Verification items for the finished model (mm, model axes). A direction names the side the tool comes from. Coordinates: 2 decimals unless noted, no trailing zeros. Order: outer loops, then holes, each group sorted by start corner. A loop starts at its lowest first (then second) coordinate and runs counter-clockwise, first axis right, second up.
Q1. Cross-section at D-D, the plane y = 9. Record the boundary of the cut face in (x, z).
Q2. Cross-section at C-C, the plane z = 15.5. Record the boundary of the cut face in (x, y).
Q3. Cross-section at B-B, the plane x = 2.5. Record the boundary of the cut face in (y, z).
Q4. Depth check by flat-ended pin: P1, Ø9.5, axis at y = 5, z = 17, coming from the +X side; P2, Ø6, axis at x = 4, y = 3, coming from the +Z side; P3, Ø10, axis at x = -4, y = -1, coming from the +Z side. Enter the tip coordinate at first touch or a pass-through.
Q5. Set-up check for faces 1 (the flat face through (-10, 6, 23.5)), 2 (the flat face through (0, -0.24, 10)): record each of +Z, -Z, +X, -X, +Y, -Y from which the full face is reachable in a straight line by a thin tool's end or side.
Q6. Cross-section at A-A, the plane y = 5.76. Record the boundary of the cut face in (x, z).
Q7. Draft check along X on faces 3 (the flat face through (-2, -3.24, 9)), 4 (the cylindrical face through (2.35, 4.24, 1.77)), 5 (the flat face through (-8.178, 5.634, 22.514)). Enter one of: pulls with the +X half, pulls with the -X half, needs draft (parallel to the pull), parting line crosses it, or undercut.
Q8. Thickness scan on line 1 (Y direction, x = 2.5, z = 11.5); line 2 (Z direction, x = 0, y = 11.5); line 3 (Z direction, x = -9.8, y = 5.76). Record the ranges inside material, lowest first.
from build123d import *

# Parameters (mm, degrees)
ESQUISSE1_W             = 23
ESQUISSE1_H             = 18
BOSS_EXTRU_1_DEPTH      = 3.5
ESQUISSE2_W             = 3.5
ESQUISSE2_H             = 18
BOSS_EXTRU_2_DEPTH      = 20
ESQUISSE3_R             = 2.5
ENL_V_MAT_EXTRU_1_DEPTH = 20
ESQUISSE4_R             = 2.5
ENL_V_MAT_EXTRU_2_DEPTH = 20
CHANFREIN1_SIZE         = 5
CHANFREIN2_SIZE         = 2
BOSS_EXTRU_3_DEPTH      = 3
BOSS_EXTRU_4_DEPTH      = 3


with BuildPart() as part:
    # Esquisse1 → Boss.-Extru.1 (new body)
    with BuildSketch(Plane.XY):
        with Locations((0.836143498, 5.76)):
            Rectangle(ESQUISSE1_W, ESQUISSE1_H)
    extrude(amount=BOSS_EXTRU_1_DEPTH)

    # Esquisse2 → Boss.-Extru.2 (add)
    with BuildSketch(Plane.XY.offset(3.5)):
        with Locations((-8.913856502, 5.76)):
            Rectangle(ESQUISSE2_W, ESQUISSE2_H)
    extrude(amount=BOSS_EXTRU_2_DEPTH)

    # Esquisse3 → Enlèv. mat.-Extru.1 (cut)
    with BuildSketch(Plane.XY.offset(3.5)):
        with Locations((4.336143498, 5.76)):
            Circle(ESQUISSE3_R)
    extrude(amount=-ENL_V_MAT_EXTRU_1_DEPTH, mode=Mode.SUBTRACT)

    # Esquisse4 → Enlèv. mat.-Extru.2 (cut)
    with BuildSketch(Plane(origin=(-7.163856502, 0, 0), x_dir=(0, 0, -1), z_dir=(1, 0, 0))):
        with Locations(Location((-15.5, 5.76, 0), (0, 0, 90))):
            Circle(ESQUISSE4_R)
    extrude(amount=-ENL_V_MAT_EXTRU_2_DEPTH, mode=Mode.SUBTRACT)

    # Chanfrein1
    chanfrein1_edges = [part.edges().sort_by_distance(p)[0] for p in [
        (-7.163856502, 5.76, 3.5),
    ]]
    chamfer(chanfrein1_edges, length=CHANFREIN1_SIZE)

    # Chanfrein2
    chanfrein2_edges = [part.edges().sort_by_distance(p)[0] for p in [
        (12.336143498, 5.76, 3.5),
        (-7.163856502, 5.76, 23.5),
    ]]
    chamfer(chanfrein2_edges, length=CHANFREIN2_SIZE)

    # Esquisse5 → Boss.-Extru.3 (add)
    with BuildSketch(Plane(origin=(0, 14.76, 0), x_dir=(1, 0, 0), z_dir=(0, 1, 0))):
        Polygon((10.336143498, -3.5), (-7.163856502, -21.5), (-7.163856502, -8.5), (-2.163856502, -3.5), align=None)
    extrude(amount=-BOSS_EXTRU_3_DEPTH)

    # Esquisse6 → Boss.-Extru.4 (add)
    with BuildSketch(Plane(origin=(0, -3.24, 0), x_dir=(-1, 0, 0), z_dir=(0, -1, 0))):
        Polygon((7.163856502, -21.5), (-10.336143498, -3.5), (2.163856502, -3.5), (7.163856502, -8.5), align=None)
    extrude(amount=-BOSS_EXTRU_4_DEPTH)


solid = part.part
Check values:
1. outline: (-10.66, 0) - (12.34, 0) - (12.34, 1.5) - (10.34, 3.5) - (-2.16, 3.5) - (-7.16, 8.5) - (-7.16, 21.5) - (-9.16, 23.5) - (-10.66, 23.5) - close
2. outline: (-10.66, -3.24) - (-1.33, -3.24) - (-1.33, -0.24) - (-7.16, -0.24) - (-7.16, 3.26) - (-10.66, 3.26) - close; (-10.66, 8.26) - (-7.16, 8.26) - (-7.16, 11.76) - (-1.33, 11.76) - (-1.33, 14.76) - (-10.66, 14.76) - close
3. outline: (-3.24, 0) - (4.06, 0) - (4.06, 3.5) - (-0.24, 3.5) - (-0.24, 11.56) - (-3.24, 11.56) - close; (7.46, 0) - (14.76, 0) - (14.76, 11.56) - (11.76, 11.56) - (11.76, 3.5) - (7.46, 3.5) - close
4. P1: stops at x = -7.16
4. P2: stops at z = 3.5
4. P3: stops at z = 23.34
5. face 1: +Z, +X, -X, +Y, -Y
5. face 2: +Z, +X
6. outline: (-10.66, 0) - (1.84, 0) - (1.84, 3.5) - (-2.16, 3.5) - (-7.16, 8.5) - (-7.16, 13) - (-10.66, 13) - close; (-10.66, 18) - (-7.16, 18) - (-7.16, 21.5) - (-9.16, 23.5) - (-10.66, 23.5) - close; (6.84, 0) - (12.34, 0) - (12.34, 1.5) - (10.34, 3.5) - (6.84, 3.5) - close
7. face 3: needs draft
7. face 4: undercut
7. face 5: pulls with the +X half
8. line 1: y = -3.24 to -0.24, 11.76 to 14.76
8. line 2: z = 0 to 3.5
8. line 3: z = 0 to 13, 18 to 23.5
